from build123d import *

# Parameters (mm, degrees)
BOSS_EXTRUDE1_DEPTH = 3.2
SKETCH11_W          = 3.2
SKETCH11_H          = 199.000000018
CUT_EXTRUDE1_DEPTH  = 284.232260808
SKETCH13_W          = 38.1
SKETCH13_H          = 38.1
CUT_EXTRUDE3_DEPTH  = 284.232260808
SKETCH15_W          = 3.175
SKETCH15_H          = 141.090166638
SKETCH15_H_2        = 141.087880638
CUT_EXTRUDE5_DEPTH  = 284.232260808


with BuildPart() as part:
    # Sketch1 → Boss-Extrude1 (new body)
    with BuildSketch(Plane(origin=(0, 0, 0), x_dir=(1, 0, 0), z_dir=(0, 1, 0))):
        Polygon((265.160373285, -60.637626629), (259.623773233, -60.637626629), (259.623773233, -62.400000041), (-255.462493265, -62.400000041), (-255.462493265, -60.637626629), (-260.999093317, -60.637626629), (-260.999093317, 99.500000009), (265.160373285, 99.500000009), align=None)
    extrude(amount=BOSS_EXTRUDE1_DEPTH)

    # Sketch11 → Cut-Extrude1 (cut, through all)
    with BuildSketch(Plane(origin=(0, 3.2, 0), x_dir=(1, 0, 0), z_dir=(0, 1, 0))):
        with Locations((2.080639984, 99.500000009)):
            Rectangle(SKETCH11_W, SKETCH11_H)
    extrude(amount=-CUT_EXTRUDE1_DEPTH, mode=Mode.SUBTRACT)

    # Sketch13 → Cut-Extrude3 (cut, through all)
    with BuildSketch(Plane(origin=(0, 3.2, 0), x_dir=(1, 0, 0), z_dir=(0, 1, 0))):
        with Locations((-18.569360016, 80.450000009)):
            Rectangle(SKETCH13_W, SKETCH13_H)
        with Locations((22.730639984, 80.450000009)):
            Rectangle(SKETCH13_W, SKETCH13_H)
    extrude(amount=-CUT_EXTRUDE3_DEPTH, mode=Mode.SUBTRACT)

    # Sketch15 → Cut-Extrude5 (cut, through all)
    with BuildSketch(Plane(origin=(0, 3.2, 0), x_dir=(1, 0, 0), z_dir=(0, 1, 0))):
        with Locations((-259.411593317, 9.90745669)):
            Rectangle(SKETCH15_W, SKETCH15_H)
        with Locations((263.572873285, 9.90631369)):
            Rectangle(SKETCH15_W, SKETCH15_H_2)
    extrude(amount=-CUT_EXTRUDE5_DEPTH, mode=Mode.SUBTRACT)


solid = part.part
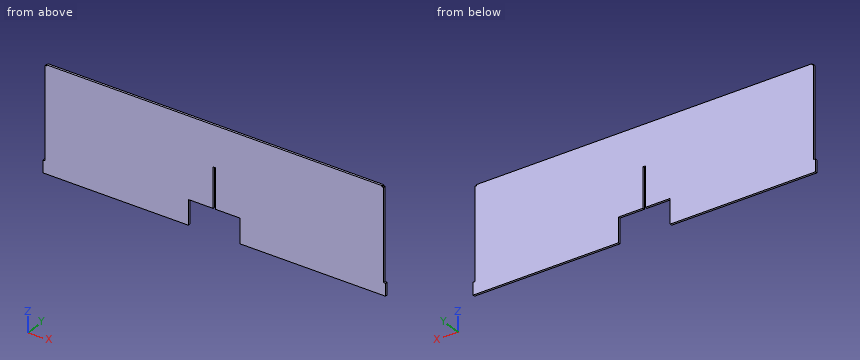
Design review of the part built by this model. Coordinates are the model's own, in mm. Coordinates: 2 decimals unless noted, no trailing zeros. Order: outer loops, then holes, each group sorted by start corner. A loop starts at its lowest first (then second) coordinate and runs counter-clockwise, first axis right, second up.
Item 1: For line 1 (X direction, y = 2.6, z = -14); line 2 (X direction, y = 1.3, z = -64); line 3 (X direction, y = 1.35, z = 27), list the stretches that pass through material, from the lowest coordinate up.
Item 2: Take a section at C-C, the plane z = -71. Write out the cut boundary in (x, y), then the cut area to 3 significant figures.
Item 3: Take a section at A-A, the plane z = -33. Write out the cut boundary in (x, y), then the cut area to 3 significant figures.
Item 4: Take a section at B-B, the plane y = 1.35. Write out the cut boundary in (x, z).
Item 5: For pin 1 Ø0.7 at (x, y) = (260.5, 1) entering from +Z; pin 2 Ø1 at (y, z) = (2.5, 6) entering from -X; pin 3 Ø1.6 at (y, z) = (1.5, 11.5) entering from +X, all flat-tipped, find the tip position at first contact; note any pin that passes through.
The answers:
1. line 1: x = -257.82 to 0.48, 3.68 to 261.99
1. line 2: x = -257.82 to -37.62, 41.78 to 261.99
1. line 3: x = -257.82 to 261.99
2. outline: (-257.82, 0) - (-37.62, 0) - (-37.62, 3.2) - (-257.82, 3.2) - close; (41.78, 0) - (261.99, 0) - (261.99, 3.2) - (41.78, 3.2) - close
2. area: 1,410 mm2
3. outline: (-257.82, 0) - (0.48, 0) - (0.48, 3.2) - (-257.82, 3.2) - close; (3.68, 0) - (261.99, 0) - (261.99, 3.2) - (3.68, 3.2) - close
3. area: 1,650 mm2
4. outline: (-261, -99.5) - (-37.62, -99.5) - (-37.62, -61.4) - (0.48, -61.4) - (0.48, 0) - (3.68, 0) - (3.68, -61.4) - (41.78, -61.4) - (41.78, -99.5) - (265.16, -99.5) - (265.16, -80.45) - (261.99, -80.45) - (261.99, 60.64) - (259.62, 60.64) - (259.62, 62.4) - (-255.46, 62.4) - (-255.46, 60.64) - (-257.82, 60.64) - (-257.82, -80.45) - (-261, -80.45) - close
5. pin 1: stops at z = 60.64
5. pin 2: stops at x = -257.82
5. pin 3: stops at x = 261.99
